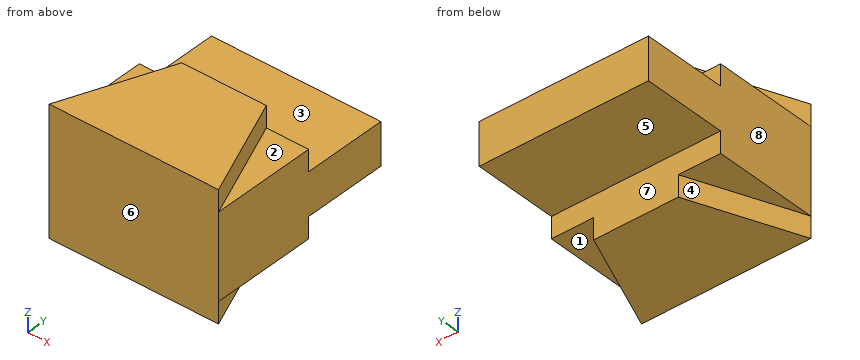
```python
from build123d import *

# Parameters (mm, degrees)
SALIENTE_EXTRUIR1_DEPTH = 20
CORTAR_EXTRUIR1_DEPTH   = 5


with BuildPart() as part:
    # Croquis1 → Saliente-Extruir1 (new, symmetric)
    with BuildSketch(Plane(origin=(0, 0, 0), x_dir=(0, 0, -1), z_dir=(1, 0, 0))):
        Polygon((-15, 0), (15, 0), (15, 25), (5, 25), (5, 45), (-5, 45), (-5, 25), (-15, 25), align=None)
    extrude(amount=SALIENTE_EXTRUIR1_DEPTH, both=True)

    # Croquis3 → Cortar-Extruir1 (cut)
    with BuildSketch(Plane.XY.offset(15)):
        Polygon((-20, 25), (-10, 25), (-20, 0), align=None)
        Polygon((10, 25), (20, 25), (20, 0), align=None)
    cortar_extruir1 = extrude(amount=-CORTAR_EXTRUIR1_DEPTH, mode=Mode.SUBTRACT)

    # Simetría1: Cortar-Extruir1 across plane
    add(cortar_extruir1.mirror(Plane.XY), mode=Mode.SUBTRACT)


solid = part.part
```
Geometry check sheet. Reference: the model listing, model coordinates, mm. Face numbers are marked on the shaded views. A direction names the side the tool comes from. Round coordinates to 2 decimals unless told otherwise and drop trailing zeros. Order: outer loops, then holes, each group sorted by start corner. A loop starts at its lowest first (then second) coordinate and runs counter-clockwise, first axis right, second up. Notation, with made-up numbers: (31, 0) - (83, 0) arc R33 cw to (83, 32) - close; hole circle Ø10 at (70, -34). An arc over 180 degrees is marked (long way). Use a Markdown table: item, result. Add a question column.
(1) Sectioned sample at B-B, the plane y = 17. Enter the section's corners in (x, z).
(2) Sectioned sample at A-A, the plane x = 16. Enter the section's corners in (y, z).
(3) Release check for a two-part mould opening along Y. For the marked faces 6, 7 and 8 record: pulls with the +Y half, pulls with the -Y half, needs draft (parallel to the pull), parting line crosses it, or undercut.
(4) Depth check by flat-ended pin: pin 1 (1.5 mm diameter, centred on y = 26, z = -7.5, fed in from +X); pin 2 (6 mm diameter, centred on x = -7, y = 33.5, fed in from -Z); pin 3 (11 mm diameter, centred on x = 8.5, z = 11.5, fed in from +Y). Enter the tip coordinate at first touch or a pass-through.
(5) Sectioned sample at C-C, the plane z = 11.25. Enter the section's corners in (x, y).
(6) Material ranges on line 1 along Y through (x, z) = (8.5, 13.5); line 2 along Z through (x, y) = (-12.5, 24); line 3 along Z through (x, y) = (-11, 37), recorded low to high. Write a range as [from, to].
(7) Tool access check on the marked faces 1, 2, 3, 4 and 5. Record the directions out of +Z, -Z, +X, -X, +Y, -Y that give a thin tool (end or side, any length) a straight path to the whole face; none if there is none.
(8) Sectioned sample at D-D, the plane x = 8. Enter the section's corners in (y, z).
Answers below:
| question | item | result |
|---|---|---|
| 1 | outline | (-20, -10) - (-13.2, -10) - (-13.2, -15) - (13.2, -15) - (13.2, -10) - (20, -10) - (20, 10) - (13.2, 10) - (13.2, 15) - (-13.2, 15) - (-13.2, 10) - (-20, 10) - close |
| 2 | outline | (0, -15) - (10, -15) - (10, -10) - (25, -10) - (25, -5) - (45, -5) - (45, 5) - (25, 5) - (25, 10) - (10, 10) - (10, 15) - (0, 15) - close |
| 3 | face 6 | pulls with the -Y half |
| 3 | face 7 | pulls with the +Y half |
| 3 | face 8 | needs draft |
| 4 | pin 1 | through |
| 4 | pin 2 | z = -5 |
| 4 | pin 3 | y = 25 |
| 5 | outline | (-20, 0) - (20, 0) - (10, 25) - (-10, 25) - close |
| 6 | line 1 | [0, 25] |
| 6 | line 2 | [-10, 10] |
| 6 | line 3 | [-5, 5] |
| 7 | face 1 | -Z, +X, +Y |
| 7 | face 2 | +Z, +X, +Y |
| 7 | face 3 | +Z, +X, -X, +Y |
| 7 | face 4 | -Z, -X, +Y |
| 7 | face 5 | -Z, +X, -X, +Y |
| 8 | outline | (0, -15) - (25, -15) - (25, -5) - (45, -5) - (45, 5) - (25, 5) - (25, 15) - (0, 15) - close |
